Answer from the drawing. Dimensions are ordinates in mm from the lowest x, y and z of the part. Round coordinates to 2 decimals unless told otherwise and drop trailing zeros. Loops run counter-clockwise (first coordinate to the right, second up) from the corner with the lowest first, then second, coordinate; pieces in that order, holes last. Notation, with made-up numbers: (40, 57.5) -> (60, 57.5) arc R18 cw to (60, 74.5) -> close; hole circle Ø6 at (0, 53.25). An arc over 180 degrees is marked (long way). Use CSV: the item, a comma, the result in double quotes. Start each with the question number.
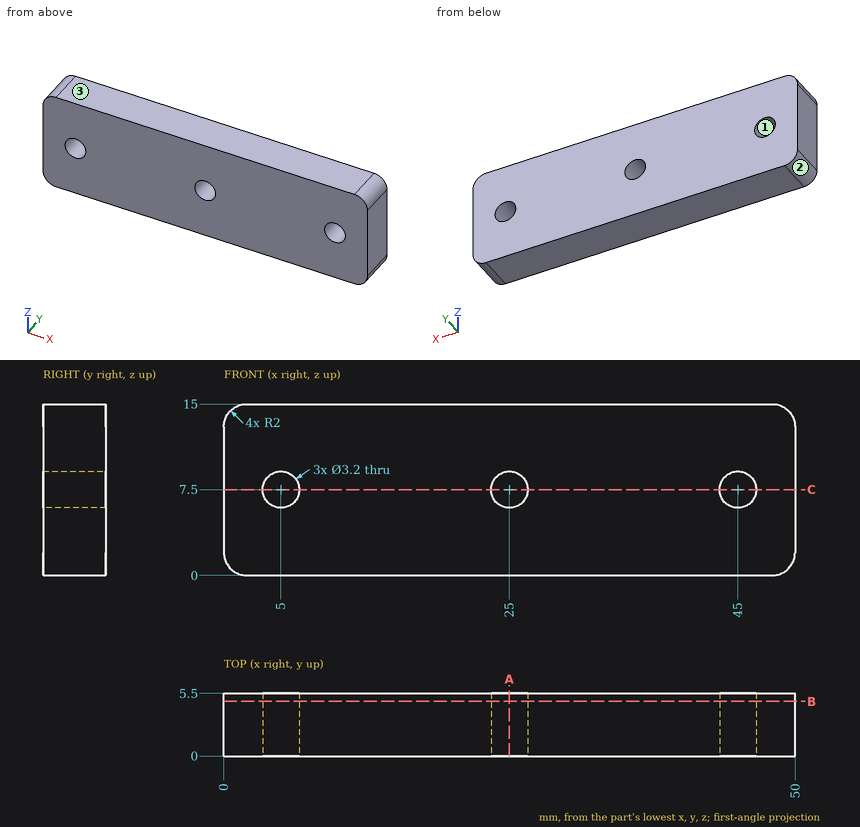
Q1. Section A-A, the plane x = 25 is taken. Write down the section's boundary in (y, z), and give its area (3 significant figures).
Q2. Straight lines are drawn through the part: line 1 (X direction, y = 3.55, z = 7.5); line 2 (X direction, y = 3.45, z = 1.5). For each, find the intervals that lie inside material, in ascending order. Write a range as from..to.
Q3. For a pull along Z with two mould halves and no side action, classify the marked faces 1, 2 and 3 as pulls with the +Z half, pulls with the -Z half, needs draft (parallel to the pull), parting line crosses it, or undercut.
Q4. Each of these flat-tipped pins is pushed along its axis until it touches: pin 1 (2.5 mm diameter, centred on x = 25, z = 7.5, fed in from -Y); pin 2 (1 mm diameter, centred on x = 20.5, y = 3.5, fed in from -Z). Where does it stop, or does it pass through?
Q5. Section C-C, the plane z = 7.5 is taken. Write down the section's boundary in (x, y).
Q6. Section B-B, the plane y = 4.8 is taken. Write down the section's boundary in (x, z).
Report:
1,outline,"(0, 0) -> (5.5, 0) -> (5.5, 5.9) -> (0, 5.9) -> close; (0, 9.1) -> (5.5, 9.1) -> (5.5, 15) -> (0, 15) -> close"
1,area,"64.9 mm²"
2,line 1,"x = 0..3.4, 6.6..23.4, 26.6..43.4, 46.6..50"
2,line 2,"x = 0.06..49.94"
3,face 1,"undercut"
3,face 2,"pulls with the -Z half"
3,face 3,"pulls with the +Z half"
4,pin 1,"passes through"
4,pin 2,"stops at z = 0"
5,outline,"(0, 0) -> (3.4, 0) -> (3.4, 5.5) -> (0, 5.5) -> close; (6.6, 0) -> (23.4, 0) -> (23.4, 5.5) -> (6.6, 5.5) -> close; (26.6, 0) -> (43.4, 0) -> (43.4, 5.5) -> (26.6, 5.5) -> close; (46.6, 0) -> (50, 0) -> (50, 5.5) -> (46.6, 5.5) -> close"
6,outline,"(0, 2) arc R2 ccw to (2, 0) -> (48, 0) arc R2 ccw to (50, 2) -> (50, 13) arc R2 ccw to (48, 15) -> (2, 15) arc R2 ccw to (0, 13) -> close; hole circle Ø3.2 at (5, 7.5); hole circle Ø3.2 at (25, 7.5); hole circle Ø3.2 at (45, 7.5)"
